For this review, take the finished solid that the model builds, in its own axes (mm). Face numbers are marked on the shaded views. A direction names the side the tool comes from. Coordinates: 2 decimals unless noted, no trailing zeros. Write each loop counter-clockwise with the first axis right and the second up, starting at its lowest first coordinate (ties: lowest second). Pieces come first, ordered by that corner, then holes. Notation, with made-up numbers: (0.25, 79.25) -> (26.25, 79.25) arc R31 cw to (26.25, 114.25) -> close; hole circle Ø1 at (-21.75, -13). An arc over 180 degrees is marked (long way). One line per item, written item: value. Start each with the question number.
1) For pin 1 Ø2.5 at (x, y) = (22.5, 22.5) entering from +Z; pin 2 Ø1.5 at (x, y) = (-22.95, -13.25) entering from +Z; pin 3 Ø2 at (y, z) = (14, -1.5) entering from -X, all flat-tipped, find the tip position at first contact; note any pin that passes through.
2) Machinability: for the marked faces 5 and 6, which of the approach directions +Z, -Z, +X, -X, +Y, -Y give a long, thin tool a straight path to every point of the face, cutting with its end or side? Answer none if there is none.
3) Mouldability with a two-part tool opening along Z and no side actions: class the marked faces 1, 2, 3 and 4 as released by +Z, released by -Z, zero draft, split by the parting line, or undercut.
4) Add section B-B (z = -16). State the section outline as (x, y) points.
5) For probe 1 along Y at (x, z) = (0, 6); probe 2 along Y at (x, z) = (0, -9); probe 3 along Z at (x, y) = (-32.5, 3), list the stretches that pass through material, from the lowest coordinate up. Write a range as from..to.
from build123d import *

# Parameters (mm, degrees)
SKETCH_1_R             = 32
EXTRUDE_1_DEPTH        = 2
SKETCH_2_R             = 30
EXTRUDE_2_DEPTH        = 8
SKETCH_3_R             = 23
CUT_EXTRUDE_1_DEPTH    = 11
SKETCH_4_R             = 26
SKETCH_4_R_2           = 23
EXTRUDE_3_DEPTH        = 23
SKETCH_5_R             = 37.5
SKETCH_5_R_2           = 1.75
SKETCH_5_R_3           = 26
SKETCH_5_R_4           = 23
EXTRUDE_4_DEPTH        = 4
HOLE_WIZARD_M4_3_D     = 3.3
HOLE_WIZARD_M4_3_DEPTH = 8.1
HOLE_WIZARD_M4_3_TIP   = 0.991420021
CHAMFER_1_SIZE         = 0.5
HOLE_WIZARD_M3_1_D     = 2.5
HOLE_WIZARD_M3_1_DEPTH = 6
HOLE_WIZARD_M3_1_TIP   = 0.751075774
CHAMFER_2_SIZE         = 0.5
CHAMFER_3_SIZE         = 0.5


with BuildPart() as part:
    # 草图1 → 凸台-拉伸1 (new body)
    with BuildSketch(Plane.XY):
        Circle(SKETCH_1_R)
    extrude(amount=EXTRUDE_1_DEPTH)

    # 草图2 → 凸台-拉伸2 (add)
    with BuildSketch(Plane.XY.offset(2)):
        Circle(SKETCH_2_R)
    extrude(amount=EXTRUDE_2_DEPTH)

    # 草图3 → 切除-拉伸1 (cut, through all)
    with BuildSketch(Plane(origin=(0, 0, 0), x_dir=(-1, 0, 0), z_dir=(0, 0, -1))):
        Circle(SKETCH_3_R)
    extrude(amount=-CUT_EXTRUDE_1_DEPTH, mode=Mode.SUBTRACT)

    # 草图4 → 凸台-拉伸3 (add)
    with BuildSketch(Plane(origin=(0, 0, 0), x_dir=(-1, 0, 0), z_dir=(0, 0, -1))):
        Circle(SKETCH_4_R)
        Circle(SKETCH_4_R_2, mode=Mode.SUBTRACT)
    extrude(amount=EXTRUDE_3_DEPTH)

    # 草图5 → 凸台-拉伸4 (add)
    with BuildSketch(Plane(origin=(0, 0, -23), x_dir=(-1, 0, 0), z_dir=(0, 0, -1))):
        Circle(SKETCH_5_R)
        with Locations((22.5, 22.5)):
            Circle(SKETCH_5_R_2, mode=Mode.SUBTRACT)
        with Locations((-22.5, 22.5)):
            Circle(SKETCH_5_R_2, mode=Mode.SUBTRACT)
        with Locations((-22.5, -22.5)):
            Circle(SKETCH_5_R_2, mode=Mode.SUBTRACT)
        with Locations((22.5, -22.5)):
            Circle(SKETCH_5_R_2, mode=Mode.SUBTRACT)
        Circle(SKETCH_5_R_3, mode=Mode.SUBTRACT)
        with Locations((22.5, 22.5)):
            Circle(SKETCH_5_R_2)
        with Locations((-22.5, 22.5)):
            Circle(SKETCH_5_R_2)
        with Locations((-22.5, -22.5)):
            Circle(SKETCH_5_R_2)
        with Locations((22.5, -22.5)):
            Circle(SKETCH_5_R_2)
        Circle(SKETCH_5_R_3)
        Circle(SKETCH_5_R_4, mode=Mode.SUBTRACT)
    extrude(amount=EXTRUDE_4_DEPTH)

    # M4 螺纹孔3
    with Locations(Plane(origin=(-22.5, -22.5, -27), x_dir=(-1, 0, 0), z_dir=(0, 0, -1))):
        with Locations((0, 0), (0, 45), (-45, 0), (-45, 45)):
            Hole(HOLE_WIZARD_M4_3_D / 2, depth=HOLE_WIZARD_M4_3_DEPTH)
            with Locations((0, 0, -(HOLE_WIZARD_M4_3_DEPTH + HOLE_WIZARD_M4_3_TIP / 2))):  # 118° drill point
                Cone(0, HOLE_WIZARD_M4_3_D / 2, HOLE_WIZARD_M4_3_TIP, mode=Mode.SUBTRACT)

    # 倒角1
    chamfer_1_edges = [part.edges().sort_by_distance(p)[0] for p in [
        (-32, 0, 0),
    ]]
    chamfer(chamfer_1_edges, length=CHAMFER_1_SIZE)

    # M3 螺纹孔1
    with Locations(Plane(origin=(0, -26.5, 10), x_dir=(1, 0, 0), z_dir=(0, 0, 1))):
        with Locations((0, 0), (22.9496732, 13.25), (22.9496732, 39.75), (0, 53), (-22.9496732, 39.75), (-22.9496732, 13.25)):
            Hole(HOLE_WIZARD_M3_1_D / 2, depth=HOLE_WIZARD_M3_1_DEPTH)
            with Locations((0, 0, -(HOLE_WIZARD_M3_1_DEPTH + HOLE_WIZARD_M3_1_TIP / 2))):  # 118° drill point
                Cone(0, HOLE_WIZARD_M3_1_D / 2, HOLE_WIZARD_M3_1_TIP, mode=Mode.SUBTRACT)

    # 倒角2
    chamfer_2_edges = [part.edges().sort_by_distance(p)[0] for p in [
        (37.5, 0, -23),
        (37.5, 0, -27),
    ]]
    chamfer(chamfer_2_edges, length=CHAMFER_2_SIZE)

    # 倒角3
    chamfer_3_edges = [part.edges().sort_by_distance(p)[0] for p in [
        (-32, 0, 2),
        (-30, 0, 10),
    ]]
    chamfer(chamfer_3_edges, length=CHAMFER_3_SIZE)


solid = part.part
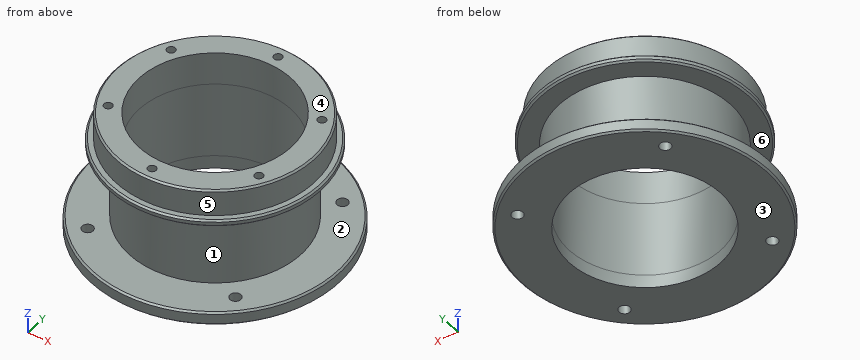
Numbers:
1. pin 1: z = 2
1. pin 2: z = 3.7
1. pin 3: x = -22.52
2. face 5: +Z
2. face 6: none
3. face 1: undercut
3. face 2: undercut
3. face 3: released by -Z
3. face 4: released by +Z
4. outline: circle Ø52 at (0, 0); hole circle Ø46 at (0, 0)
5. probe 1: -30..-27.75, -25.25..-23, 23..25.25, 27.75..30
5. probe 2: -26..-23, 23..26
5. probe 3: -27..-23
